Autodesk Inventor part; units mm, degrees
ref_plane "YZ Plane" through (0, 0, 0) normal (1, 0, 0) x (0, 1, 0)
ref_plane "XZ Plane" through (0, 0, 0) normal (0, 1, 0) x (-1, 0, 0)
ref_plane "XY Plane" through (0, 0, 0) normal (0, 0, 1) x (1, 0, 0)
sketch "Szkic1" plane through (0, 0, 0) normal (0, 1, 0) x (-1, 0, 0)
  line L0 (0, 0) -> (-100, 0)
  line L1 (-100, 0) -> (-100, -100)
  line L2 (-100, -100) -> (0, -100)
  line L3 (0, -100) -> (0, 0)
  dimension "d0" = 100
  dimension "d1" = 100
extrude "Wyciągnięcie proste1" add sketch "Szkic1" along normal blind 10
sketch "Szkic2" plane through (100, 0, -100) normal (0, 0, -1) x (-1, 0, 0)
  line L0 (0, 0) -> (5, 0)
  line L1 (5, 0) -> (15, 10)
  line L2 (0, 10) -> (100, 10)
  line L3 (5, 0) -> (19.1421, 0) construction
  line L4 (15, 10) -> (0, 10)
  line L5 (0, 10) -> (0, 0.5914)
  line L6 (0, 0) -> (100, 0)
  line L7 (0, 0.5914) -> (0, 0)
  line L8 (0, 0) -> (5, 0)
  dimension "d4" = 5
  dimension "d5" = 45
extrude "Wyciągnięcie proste2" cut sketch "Szkic2" against normal blind 100
sketch "Szkic4" plane through (0, 0, 0) normal (0, 0, 1) x (1, 0, 0)
  line L0 (0, 0) -> (100, 0)
  line L1 (100, 0) -> (100, 2)
  line L2 (100, 2) -> (0, 2)
  line L3 (0, 2) -> (0, 0)
  dimension "d8" = 100
  dimension "d9" = 2
extrude "Wyciągnięcie proste3" cut sketch "Szkic4" against normal blind 100
sketch "Szkic5" plane through (0, 10, 0) normal (0, 1, 0) x (1, 0, 0)
  line L0 (0, 0) -> (85, 0)
  line L1 (0, 0) -> (35, 0)
  line L2 (35, 0) -> (35, 15)
  line L3 (35, 15) -> (0, 15)
  line L4 (0, 15) -> (0, 0)
  line L5 (0, 100) -> (0, 0)
  line L6 (0, 100) -> (35, 100)
  line L7 (35, 100) -> (35, 85)
  line L8 (35, 85) -> (0, 85)
  line L9 (0, 85) -> (0, 100)
  dimension "d12" = 35
  dimension "d13" = 15
  dimension "d14" = 35
  dimension "d15" = 15
extrude "Wyciągnięcie proste4" cut sketch "Szkic5" against normal blind 100 contours L5 L6 L7 L8
sketch "Szkic6" plane through (0, 10, 0) normal (0, 1, 0) x (1, 0, 0)
  line L0 (0, 0) -> (93, 0)
  line L1 (0, 0) -> (35, 0)
  line L2 (35, 0) -> (35, 15)
  line L3 (35, 15) -> (0, 15)
  line L4 (0, 15) -> (0, 0)
  dimension "d18" = 35
  dimension "d19" = 15
extrude "Wyciągnięcie proste5" cut sketch "Szkic6" against normal blind 100
sketch "Szkic7" plane through (35, 2, 0) normal (0, 0, 1) x (1, 0, 0)
  line L0 (58, 0) -> (50, 8)
  line L1 (58, 0) -> (-42, 0)
  line L2 (-42, 0) -> (-42, 2)
  line L3 (-42, 2) -> (58, 2)
  line L4 (58, 2) -> (58, 0)
  point P0 (-35, -2)
  point P1 (56, 2)
  dimension "d22" = 100
  dimension "d23" = 2
extrude "Wyciągnięcie proste6" cut sketch "Szkic7" against normal blind 101.5 contours L1 L2 L3 L0
sketch "Szkic8" plane through (0, 10, 0) normal (0, 1, 0) x (1, 0, 0)
  line L0 (83, 93) -> (75.5, 93)
  line L1 (75.5, 93) -> (75.5, 85.5)
  line L2 (75.5, 85.5) -> (83, 85.5)
  line L3 (83, 85.5) -> (83, 93)
  point P0 (0, 0)
  dimension "d26" = 7.5
  dimension "d27" = 7.5
extrude "Wyciągnięcie proste7" cut sketch "Szkic8" against normal blind 10
sketch "Szkic9" plane through (0, 10, 0) normal (0, 1, 0) x (1, 0, 0)
  line L0 (83, 7) -> (75.5, 7)
  line L1 (75.5, 7) -> (75.5, 14.5)
  line L2 (75.5, 14.5) -> (83, 14.5)
  line L3 (83, 14.5) -> (83, 7)
  point P0 (0, 0)
  dimension "d30" = 7.5
  dimension "d31" = 7.5
extrude "Wyciągnięcie proste8" cut sketch "Szkic9" against normal blind 10
sketch "Szkic11" plane through (35, 10, 0) normal (0, 0, 1) x (1, 0, 0)
  line L0 (0, -6) -> (56, -6)
  line L1 (-35, 0) -> (-35, -6)
  line L2 (56, -6) -> (-35, -6)
  line L3 (-35, -6) -> (-35, -5)
  line L4 (-35, -5) -> (56, -5)
  line L5 (56, -5) -> (56, -6)
  point P0 (-35, -10)
  dimension "d34" = 1
extrude "Wyciągnięcie proste9" cut sketch "Szkic11" against normal blind 100.75
properties part number "Helenowiak_podstawa"
Input: part model. Units: mm. Frame: model coordinates. A direction names the side the tool comes from. Round coordinates to 2 decimals unless told otherwise and drop trailing zeros. Order: outer loops, then holes, each group sorted by start corner. A loop starts at its lowest first (then second) coordinate and runs counter-clockwise, first axis right, second up. Notation, with made-up numbers: (10.25, 78.25) - (25.25, 78.25) arc R23 ccw to (25.25, 94.25) - close; hole circle Ø9 at (19.25, 55.5). An arc over 180 degrees is marked (long way). Answer in a Markdown table with one row per item.
Item 1: Line query: line 1 (Z direction, x = 15, y = 8.4); line 2 (X direction, y = 5.6, z = -76); line 3 (X direction, y = 8.5, z = -49). Output: solid intervals per line, ascending.
Model answer:
| item | result |
|---|---|
| line 1 | z = -85 to -15 |
| line 2 | x = 0 to 89.4 |
| line 3 | x = 0 to 86.5 |
Item 2: Pin query (flat end, axial travel): pin 1 (1.5 mm diameter, centred on x = 21, y = 8.5, fed in from +Z); pin 2 (1.5 mm diameter, centred on x = 21.5, y = 8.5, fed in from -Z); pin 3 (2.5 mm diameter, centred on y = 8.5, z = -9, fed in from +X); pin 4 (1.5 mm diameter, centred on y = 8.5, z = -32, fed in from -X). Return the tip coordinate at first contact, or that it passes through.
Model answer:
| item | result |
|---|---|
| pin 1 | stops at z = -15 |
| pin 2 | stops at z = -85 |
| pin 3 | stops at x = 87.75 |
| pin 4 | stops at x = 0 |
Item 3: Section query B-B (y = 6.3). Return the cut outline in (x, z).
Model answer:
| item | result |
|---|---|
| outline | (0, -85) - (35, -85) - (35, -100) - (88.7, -100) - (88.7, 0) - (35, 0) - (35, -15) - (0, -15) - close; hole (75.5, -93) - (83, -93) - (83, -85.5) - (75.5, -85.5) - close; hole (75.5, -14.5) - (83, -14.5) - (83, -7) - (75.5, -7) - close |
Item 4: Section query A-A (x = 77.5). Return the cut outline in (y, z), then the cut area to 3 significant figures.
Model answer:
| item | result |
|---|---|
| outline | (5, -100) - (10, -100) - (10, -93) - (5, -93) - close; (5, -85.5) - (10, -85.5) - (10, -14.5) - (5, -14.5) - close; (5, -7) - (10, -7) - (10, 0) - (5, 0) - close |
| area | 425 mm² |
Item 5: Reachability of faces 1 (the flat face through (63, 7, -100)), 2 (the flat face through (0, 7, -50)), 3 (the flat face through (18, 8, -85)), 4 (the flat face through (75.5, 8, -11)), 5 (the flat face through (35, 8, -7)) from +Z, -Z, +X, -X, +Y, -Y: full face, straight path, thin tool, end or side. Return the list, or none.
Model answer:
| item | result |
|---|---|
| face 1 | -Z, +X, -X, +Y, -Y |
| face 2 | +Z, -Z, -X, +Y, -Y |
| face 3 | -Z, -X, +Y, -Y |
| face 4 | +Y, -Y |
| face 5 | +Z, -X, +Y, -Y |
Item 6: Mould query, pull axis X, two halves, no side actions, for faces 6 (the flat face through (18, 8, -15)), 7 (the flat face through (83, 8, -11)), 8 (the flat face through (35, 8, -93)). Classes: released by +X, released by -X, zero draft, split by the parting line, or undercut.
Model answer:
| item | result |
|---|---|
| face 6 | zero draft |
| face 7 | undercut |
| face 8 | released by -X |
Item 7: Section query D-D (x = 9). Return the cut outline in (y, z).
Model answer:
| item | result |
|---|---|
| outline | (5, -85) - (10, -85) - (10, -15) - (5, -15) - close |
Item 8: Section query C-C (z = -30.5). Return the cut outline in (x, y), then the cut area to 4 significant figures.
Model answer:
| item | result |
|---|---|
| outline | (0, 5) - (90, 5) - (85, 10) - (0, 10) - close |
| area | 437.5 mm² |
